```python
from build123d import *

# Parameters (mm, degrees)
F0_R     = 25
F1_DEPTH = 75
F2_T     = -0.4
F3_W     = 30
F3_H     = 26
F4_DEPTH = 25.001


with BuildPart() as f1:
    # F0 (on Top) → F1 (new body)
    with BuildSketch(Plane.XY):
        Circle(F0_R)
    extrude(amount=F1_DEPTH)

    # F2
    f2_openings = [f1.faces().sort_by_distance(p)[0] for p in [
        (0, 0, 75),
    ]]
    offset(amount=F2_T, openings=f2_openings)

    # F3 (on Front) → F4 (cut, through all)
    with BuildSketch(Plane.XZ):
        with Locations((0, 62)):
            Rectangle(F3_W, F3_H)
    extrude(amount=-F4_DEPTH, mode=Mode.SUBTRACT)


solid = f1.part
```
Work out the finished part from the listing and answer in its coordinate system (mm). Round coordinates to 2 decimals unless told otherwise and drop trailing zeros. Write each loop counter-clockwise with the first axis right and the second up, starting at its lowest first coordinate (ties: lowest second). Pieces come first, ordered by that corner, then holes.
1) A cutting plane is placed at A-A on y = 0. Determine the outline of the cut face in (x, z).
2) A cutting plane is placed at D-D on z = 67.5. Determine the outline of the cut face in (x, y), and give its area (3 significant figures).
3) A cutting plane is placed at C-C on x = 0. Determine the outline of the cut face in (y, z).
4) Flat-ended cylindrical pins translate along their axes: P1, Ø6, axis at x = -1.5, z = 13, coming from the +Y side; P2, Ø4, axis at x = -17, z = 58, coming from the -Y side; P3, Ø4, axis at x = 2, z = 29.5, coming from the -Y side. Find the tip coordinate at first contact, or state that the pin passes through.
5) Consider probe 1 along Y at (x, z) = (0, 43.5); probe 2 along Z at (x, y) = (-15, -1.5). Determine where each line is inside the solid, lowest interval first.
6) A cutting plane is placed at B-B on z = 5.5. Determine the outline of the cut face in (x, y).
7) Determine the mould class of faces 1 (the face through (-5.42, -24.406, 36.975)), 2 (the face through (-5.7, -24.1, 75)), 3 (the face through (0, 0, 0.4)), 4 (the face through (-5.333, -24.015, 37.178)) for opening direction Y: pulls with the +Y half, pulls with the -Y half, needs draft (parallel to the pull), parting line crosses it, or undercut.
Entries:
1. outline: (-25, 0) - (25, 0) - (25, 75) - (24.6, 75) - (24.6, 0.4) - (-24.6, 0.4) - (-24.6, 75) - (-25, 75) - close
2. outline: (-15, 19.5) - (-15, 20) arc R25 ccw (long way) to (15, 20) - (15, 19.5) arc R24.6 cw (long way) to start
2. area: 49.4 mm2
3. outline: (-25, 0) - (25, 0) - (25, 49) - (24.6, 49) - (24.6, 0.4) - (-24.6, 0.4) - (-24.6, 75) - (-25, 75) - close
4. P1: stops at y = 25
4. P2: stops at y = -20
4. P3: stops at y = -25
5. probe 1: y = -25 to -24.6, 24.6 to 25
5. probe 2: z = 0 to 0.4
6. outline: circle Ø50 at (0, 0); hole circle Ø49.2 at (0, 0)
7. face 1: parting line crosses it
7. face 2: needs draft
7. face 3: undercut
7. face 4: undercut
